from build123d import *

# Parameters (mm, degrees)
F0_W     = 19.05
F0_H     = 44.45
F1_DEPTH = 25.4
F2_W     = 12.7
F2_H     = 44.45
F3_DEPTH = 25.4
F5_DEPTH = 25.4
F6_W     = 12.7
F6_H     = 44.45
F7_DEPTH = 31.75
F8_R     = 9.525
F9_DEPTH = 25.4


with BuildPart() as f1:
    # F0 (on Front) → F1 (new body)
    with BuildSketch(Plane.XZ):
        with Locations((-54.87412, 22.225)):
            Rectangle(F0_W, F0_H)
    extrude(amount=F1_DEPTH)

    # F2 (on face) → F3 (join)
    with BuildSketch(Plane.YZ.offset(-45.34912)):
        with Locations((-19.05, 22.225)):
            Rectangle(F2_W, F2_H)
    extrude(amount=F3_DEPTH)

    # F4 (on face) → F5 (cut)
    with BuildSketch(Plane(origin=(0, -12.7, 0), x_dir=(-1, 0, 0), z_dir=(0, 1, 0))):
        Polygon((19.94912, 0), (45.34912, 44.45), (19.94912, 44.45), align=None)
    extrude(amount=-F5_DEPTH, mode=Mode.SUBTRACT)

    # F6 (on face) → F7 (join)
    with BuildSketch(Plane.YZ.offset(-45.34912)):
        with Locations((-6.35, 22.225)):
            Rectangle(F6_W, F6_H)
    extrude(amount=F7_DEPTH)

    # F8 (on face) → F9 (cut)
    with BuildSketch(Plane(origin=(0, 0, 0), x_dir=(-1, 0, 0), z_dir=(0, 1, 0))):
        with Locations((42.17412, 25.4)):
            Circle(F8_R)
    extrude(amount=-F9_DEPTH, mode=Mode.SUBTRACT)


solid = f1.part
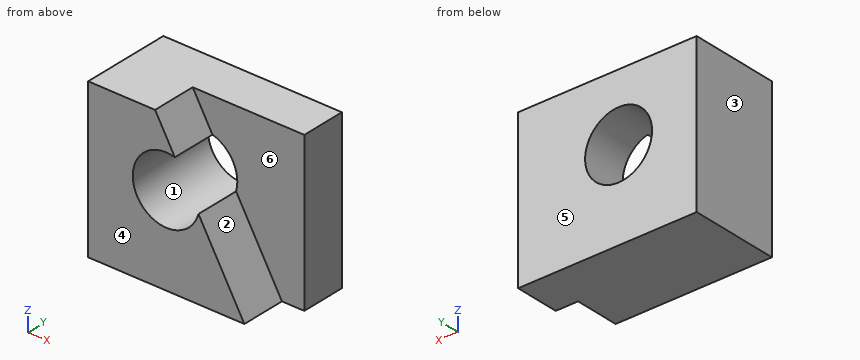
Can you work these out from the model? Positions are in its coordinate system, mm. Face numbers are marked on the shaded views. A direction names the side the tool comes from. Coordinates: 2 decimals unless noted, no trailing zeros. Loops run counter-clockwise (first coordinate to the right, second up) from the corner with the lowest first, then second, coordinate; pieces in that order, holes last. Notation, with made-up numbers: (12.25, -29) - (36.25, -29) arc R20 ccw to (36.25, -15) - close; hole circle Ø2 at (-23, -26.75). An arc over 180 degrees is marked (long way). Answer as a JSON object with one key per item and string values. Group by question number.
Item 1: On a 3-axis mill with a long thin cutter (end or side, diameter ignored), from which of +Z, -Z, +X, -X, +Y, -Y can I reach the whole of each face in a straight line? I mean the marked faces 5 and 6. Say none if no direction works.
Item 2: If I drill on L1, parallel to Y at x = -23.5, z = 11.5; L2, parallel to X at y = -6.5, z = 25.4; L3, parallel to X at y = -19.75, z = 25.4, over which ranges is the centre line in solid material (lowest first)? Write a range as from..to.
Item 3: If we section it at D-D (y = -15.5): List the corners of the cut face in (x, z) for me (3 decimals).
Item 4: If we section it at C-C (y = -4.25): List the corners of the cut face in (x, z) for me (3 decimals).
Item 5: If we mould it in two halves opening along X, with no side actions, what happens to the marked faces 1, 2, 3 and 4? For each: released by +X, released by -X, zero draft, split by the parting line, or undercut.
Item 6: For pin 1 (2 mm diameter, centred on x = -23.5, z = 39, fed in from -Y), with a flat end and sliding along its axis, tell me the tip position at first contact or that it passes through.
Item 7: If we section it at A-A (z = 25.4): List the corners of the cut face in (x, y) for me.
Item 8: If we section it at B-B (x = -38): List the corners of the cut face in (y, z) for me, plus the area to 3 significant figures.
Returned:
{
 "1": {"face 5": "+Z, -Z, +X, -X, +Y", "face 6": "+Z, +X, -Y"},
 "2": {"L1": "y = -12.7..0", "L2": "x = -64.4..-51.7, -32.65..-13.6", "L3": "x = -64.4..-51.7"},
 "3": {"outline": "(-64.399, 0) - (-19.949, 0) - (-33, 22.839) arc R9.525 cw (long way) to (-39.723, 34.604) - (-45.349, 44.45) - (-64.399, 44.45) - close"},
 "4": {"outline": "(-64.399, 0) - (-13.599, 0) - (-13.599, 44.45) - (-64.399, 44.45) - close; hole circle Ø19.05 at (-42.174, 25.4)"},
 "5": {"face 1": "undercut", "face 2": "released by +X", "face 3": "released by -X", "face 4": "zero draft"},
 "6": {"pin 1": "stops at y = -12.7"},
 "7": {"outline": "(-64.4, -25.4) - (-51.7, -25.4) - (-51.7, 0) - (-64.4, 0) - close; (-32.65, -12.7) - (-13.6, -12.7) - (-13.6, 0) - (-32.65, 0) - close"},
 "8": {"outline": "(-25.4, 0) - (0, 0) - (0, 16.84) - (-25.4, 16.84) - close; (-12.7, 33.96) - (0, 33.96) - (0, 44.45) - (-12.7, 44.45) - close", "area": "561 mm²"}
}
